Check sheet for the drawn part. Datum: minimum x, y, z corner. Units: mm. Round coordinates to 2 decimals unless told otherwise and drop trailing zeros. Order: outer loops, then holes, each group sorted by start corner. A loop starts at its lowest first (then second) coordinate and runs counter-clockwise, first axis right, second up. Notation, with made-up numbers: (16, 4) -> (64, 4) arc R21 ccw to (64, 22) -> close; hole circle Ø1 at (-22, -32). An arc over 180 degrees is marked (long way). Answer in a Markdown table with one row per item.
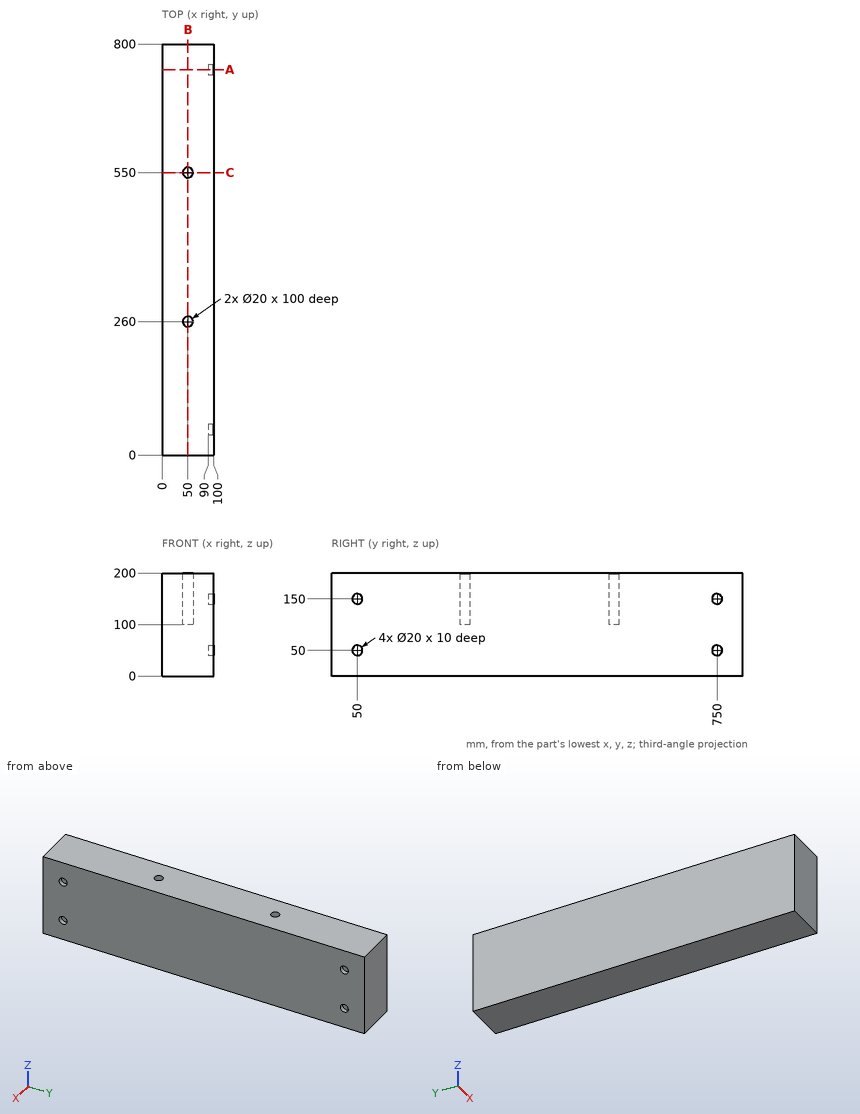
(1) Depth check by flat-ended pin: pin 1 Ø4 at (x, y) = (66.5, 547) entering from -Z; pin 2 Ø6 at (y, z) = (747.5, 145.5) entering from +X; pin 3 Ø16 at (x, y) = (50, 260) entering from +Z. Enter the tip coordinate at first touch or a pass-through.
Solutions:
| item | result |
|---|---|
| pin 1 | z = 0 |
| pin 2 | x = 90 |
| pin 3 | z = 100 |
(2) Section check B-B on x = 50. Record the boundary of the cut face in (y, z), plus the area to 3 significant figures.
Solutions:
| item | result |
|---|---|
| outline | (0, 0) -> (800, 0) -> (800, 200) -> (560, 200) -> (560, 100) -> (540, 100) -> (540, 200) -> (270, 200) -> (270, 100) -> (250, 100) -> (250, 200) -> (0, 200) -> close |
| area | 156,000 mm^2 |
(3) Section check A-A on y = 750. Record the boundary of the cut face in (x, z), plus the area to 3 significant figures.
Solutions:
| item | result |
|---|---|
| outline | (0, 0) -> (100, 0) -> (100, 40) -> (90, 40) -> (90, 60) -> (100, 60) -> (100, 140) -> (90, 140) -> (90, 160) -> (100, 160) -> (100, 200) -> (0, 200) -> close |
| area | 19,600 mm^2 |
(4) Scan lines: probe 1 along Z at (x, y) = (97, 50); probe 2 along Y at (x, z) = (50, 128); probe 3 along X at (y, z) = (550, 142). Record each from-to range of solid material in increasing order. Write a range as from..to.
Solutions:
| item | result |
|---|---|
| probe 1 | 0..40, 60..140, 160..200 |
| probe 2 | 0..250, 270..540, 560..800 |
| probe 3 | 0..40, 60..100 |
(5) Section check C-C on y = 550. Record the boundary of the cut face in (x, z), plus the area to 3 significant figures.
Solutions:
| item | result |
|---|---|
| outline | (0, 0) -> (100, 0) -> (100, 200) -> (60, 200) -> (60, 100) -> (40, 100) -> (40, 200) -> (0, 200) -> close |
| area | 18,000 mm^2 |
